```python
from build123d import *

# Parameters (mm, degrees)
F0_R     = 18.5
F1_DEPTH = 22
F2_R     = 15
F3_DEPTH = 45
F4_R     = 6
F5_DEPTH = 7
F6_R     = 3
F7_DEPTH = 13


with BuildPart() as f1:
    # F0 (on Top) → F1 (new body)
    with BuildSketch(Plane.XY):
        Circle(F0_R)
    extrude(amount=F1_DEPTH)

    # F2 (on face) → F3 (join)
    with BuildSketch(Plane(origin=(0, 0, 0), x_dir=(1, 0, 0), z_dir=(0, 0, -1))):
        Circle(F2_R)
    extrude(amount=F3_DEPTH)

    # F4 (on face) → F5 (join)
    with BuildSketch(Plane.XY.offset(22)):
        with Locations((0, 8)):
            Circle(F4_R)
    extrude(amount=F5_DEPTH)

    # F6 (on face) → F7 (join)
    with BuildSketch(Plane.XY.offset(29)):
        with Locations((0, 8)):
            Circle(F6_R)
    extrude(amount=F7_DEPTH)


solid = f1.part
```
Work out the finished part from the listing and answer in its coordinate system (mm). A direction names the side the tool comes from. Round coordinates to 2 decimals unless told otherwise and drop trailing zeros. Order: outer loops, then holes, each group sorted by start corner. A loop starts at its lowest first (then second) coordinate and runs counter-clockwise, first axis right, second up.
Q1. A tool of negligible diameter and unlimited length cuts with its end or side. For faces 1 (the flat face through (0, 0, -45)), 2 (the cylindrical face through (-14.985, -0.66, -22.185)), 3 (the cylindrical face through (-1.301, 2.143, 25.451)), from which of +Z, -Z, +X, -X, +Y, -Y can it reach the whole face along a straight path? Write none if from no direction.
Solution:
face 1: -Z, +X, -X, +Y, -Y
face 2: -Z
face 3: +Z
Q2. Find the intervals of material crossed by line 1 along Z through (x, y) = (-6, -3); line 2 along Z through (x, y) = (-0.5, 11); line 3 along Y through (x, z) = (11, -10.5), in increasing order.
Solution:
line 1: z = -45 to 22
line 2: z = -45 to 29
line 3: y = -10.2 to 10.2
Q3. A cutting plane is placed at C-C, the plane z = 11.5. Determine the outline of the cut face in (x, y).
Solution:
outline: circle Ø37 at (0, 0)
Q4. A cutting plane is placed at A-A, the plane x = 0. Determine the outline of the cut face in (y, z), then the cut area to 3 significant figures.
Solution:
outline: (-18.5, 0) - (-15, 0) - (-15, -45) - (15, -45) - (15, 0) - (18.5, 0) - (18.5, 22) - (14, 22) - (14, 29) - (11, 29) - (11, 42) - (5, 42) - (5, 29) - (2, 29) - (2, 22) - (-18.5, 22) - close
area: 2,330 mm2
Q5. Given pin 1 Ø4 at (x, z) = (-12.5, 1.5) entering from -Y; pin 2 Ø11 at (x, y) = (8.5, 9) entering from +Z; pin 3 Ø5 at (x, z) = (8.5, -34) entering from +Y, each flat-ended and moving along its own axis, determine where each tip first touches the part or whether it passes through.
Solution:
pin 1: stops at y = -15.23
pin 2: stops at z = 29
pin 3: stops at y = 13.75
Q6. A cutting plane is placed at B-B, the plane y = 0. Determine the outline of the cut face in (x, z), then the cut area to 3 significant figures.
Solution:
outline: (-18.5, 0) - (-15, 0) - (-15, -45) - (15, -45) - (15, 0) - (18.5, 0) - (18.5, 22) - (-18.5, 22) - close
area: 2,160 mm2
Q7. A cutting plane is placed at D-D, the plane y = -10.5. Determine the outline of the cut face in (x, z), then the cut area to 3 significant figures.
Solution:
outline: (-15.23, 0) - (-10.71, 0) - (-10.71, -45) - (10.71, -45) - (10.71, 0) - (15.23, 0) - (15.23, 22) - (-15.23, 22) - close
area: 1,630 mm2
